from build123d import *

# Parameters (mm, degrees)
TAP_DRILL_FOR_M2_5X0_45_TAP2_D = 2.05
CUT_EXTRUDE1_DEPTH             = 21


with BuildPart() as part:
    # Sketch3 → Revolve1 (revolve)
    with BuildSketch(Plane.XY, mode=Mode.PRIVATE) as revolve1_sk:
        Polygon((-2.25, 34.3), (0, 34.3), (0, 0), (-6, 0), (-6, 32.3), (-10.5, 32.3), (-10.5, 37.15), (-14, 37.15), (-14, 40), (-4, 40), (-4, 37.15), (-2.25, 37.15), align=None)
    revolve(revolve1_sk.sketch.rotate(Axis((0, 0, 0), (0, 1, 0)), 270), axis=Axis((0, 0, 0), (0, 1, 0)))

    # Tap Drill for M2.5x0.45 Tap2 (through all)
    with Locations(Plane.XZ.offset(-32.3)):
        with Locations((-5.656854249, 5.656854249), (0, 8), (5.656854249, 5.656854249), (8, 0), (5.656854249, -5.656854249), (0, -8), (-5.656854249, -5.656854249), (-8, 0)):
            Hole(TAP_DRILL_FOR_M2_5X0_45_TAP2_D / 2)

    # Sketch13 → Cut-Extrude1 (cut)
    with BuildSketch(Plane.XZ):
        Polygon((-64.283224073, 5.196152423), (-3, 5.196152423), (3, 5.196152423), (64.283224073, 5.196152423), (64.283224073, 127.762600569), (-64.283224073, 127.762600569), align=None)
    extrude(amount=-CUT_EXTRUDE1_DEPTH, mode=Mode.SUBTRACT)


solid = part.part
The listing builds one solid part. Answer for the finished solid, in the listing's coordinates (mm). A direction names the side the tool comes from. Coordinates: 2 decimals unless noted, no trailing zeros. Loops run counter-clockwise (first coordinate to the right, second up) from the corner with the lowest first, then second, coordinate; pieces in that order, holes last.
1) Find section A-A on x = 0. Give the number of separate pieces and of enclosed holes in the cut face, then the cut area to 3 significant figures.
2) Flat-ended cylindrical pins translate along their axes: pin 1 Ø2.5 at (x, z) = (0, -8) entering from +Y; pin 2 Ø12 at (x, y) = (6, 22) entering from +Z; pin 3 Ø5 at (x, y) = (-6.5, 28) entering from -Z; pin 4 Ø4 at (x, y) = (-4.5, 32) entering from -Z. Find the tip coordinate at first contact, or state that the pin passes through.
3) Find section C-C on z = 8. Write down the section's boundary in (x, y) (3 decimals), then the cut area to 3 significant figures.
4) Find section D-D on y = 4. Write down the section's boundary in (x, z).
5) A tool of negligible diameter and unlimited length cuts with its end or side. For faces 1 (the face through (-3.2, 34.8, -10)), 2 (the face through (0.76, 36.2, 8.69)), 3 (the face through (2, 37.15, -2)), from which of +Z, -Z, +X, -X, +Y, -Y can it reach the whole face along a straight path? Write none if from no direction.
6) Determine the mould class of faces 4 (the face through (-1.802, 16.376, -5.723)), 5 (the face through (0, 10, 5.196)), 6 (the face through (-5.52, 36.2, -4.64)) for opening direction X: pulls with the +X half, pulls with the -X half, needs draft (parallel to the pull), parting line crosses it, or undercut.
7) Find section B-B on z = 0. Write down the section's boundary in (x, y) (3 decimals), then the cut area to 3 significant figures.
8) Find the intervals of material crossed by L1, parallel to Z at x = 6.5, y = 35.5; L2, parallel to Y at x = -6.75, z = 4.75; L3, parallel to Y at x = 10.5, z = -3, in increasing order.
Values:
1. separate pieces: 3
1. enclosed holes: 0
1. area: 485 mm2
2. pin 1: stops at y = 40
2. pin 2: stops at z = 6
2. pin 3: stops at z = -4.47
2. pin 4: stops at z = -10.19
3. outline: (-11.489, 37.15) - (-6.801, 37.15) - (-6.801, 32.3) - (-1.025, 32.3) - (-1.025, 40) - (-11.489, 40) - close; (1.025, 32.3) - (6.801, 32.3) - (6.801, 37.15) - (11.489, 37.15) - (11.489, 40) - (1.025, 40) - close
3. area: 116 mm2
4. outline: (-3, 5.2) arc R6 ccw (long way) to (3, 5.2) - close
5. face 1: -Y
5. face 2: +Y, -Y
5. face 3: +Y
6. face 4: parting line crosses it
6. face 5: needs draft
6. face 6: undercut
7. outline: (-14, 37.15) - (-10.5, 37.15) - (-10.5, 32.3) - (-9.025, 32.3) - (-9.025, 40) - (-14, 40) - close; (-6.975, 32.3) - (-6, 32.3) - (-6, 0) - (6, 0) - (6, 32.3) - (6.975, 32.3) - (6.975, 40) - (4, 40) - (4, 37.15) - (2.25, 37.15) - (2.25, 34.3) - (-2.25, 34.3) - (-2.25, 37.15) - (-4, 37.15) - (-4, 40) - (-6.975, 40) - close; (9.025, 32.3) - (10.5, 32.3) - (10.5, 37.15) - (14, 37.15) - (14, 40) - (9.025, 40) - close
7. area: 502 mm2
8. L1: z = -8.25 to -6.24, -5.07 to 5.07, 6.24 to 8.25
8. L2: y = 32.3 to 40
8. L3: y = 37.15 to 40
